Could you check a few things on this drawing? It's one solid part, dimensions in mm from its lowest x, y, z. A direction names the side the tool comes from. Coordinates: 2 decimals unless noted, no trailing zeros. Loops run counter-clockwise (first coordinate to the right, second up) from the corner with the lowest first, then second, coordinate; pieces in that order, holes last.
1) Imagine slicing it at C-C on y = 39. Please give me the cut outline in (x, z), plus the area to 3 significant figures.
2) Will these pins go through, and if not, where does the flat tip stop? P1, Ø7, axis at y = 50, z = 15, coming from the +X side; P2, Ø10, axis at x = 19.5, z = 7, coming from the +Y side; P3, Ø14.5, axis at x = 15, y = 15, coming from the -Z side; P4, Ø12, axis at x = 14.5, z = 9, coming from the +Y side.
3) Imagine slicing it at A-A on z = 15. Please give me the cut outline in (x, y), plus the area to 3 significant figures.
4) Imagine slicing it at D-D on z = 2.25. Please give me the cut outline in (x, y), plus the area to 3 significant figures.
5) Imagine slicing it at B-B on x = 15. Please give me the cut outline in (y, z), plus the area to 3 significant figures.
6) Thinking about a two-plate mould opening in Z: for the marked faces 1, 2, 3 and 4, which applies, released by +Z, released by -Z, zero draft, split by the parting line, or undercut?
7) For the marked faces 5 and 6, which set-ups out of +Z, -Z, +X, -X, +Y, -Y let a thin tool reach every point of the face, with its end or its side?
8) If I drill on line 1 along X through (y, z) = (54, 8.5); line 2 along Z through (x, y) = (2.5, 50); line 3 along Y through (x, z) = (16.5, 22.75), over which ranges is the centre line in solid material (lowest first)?
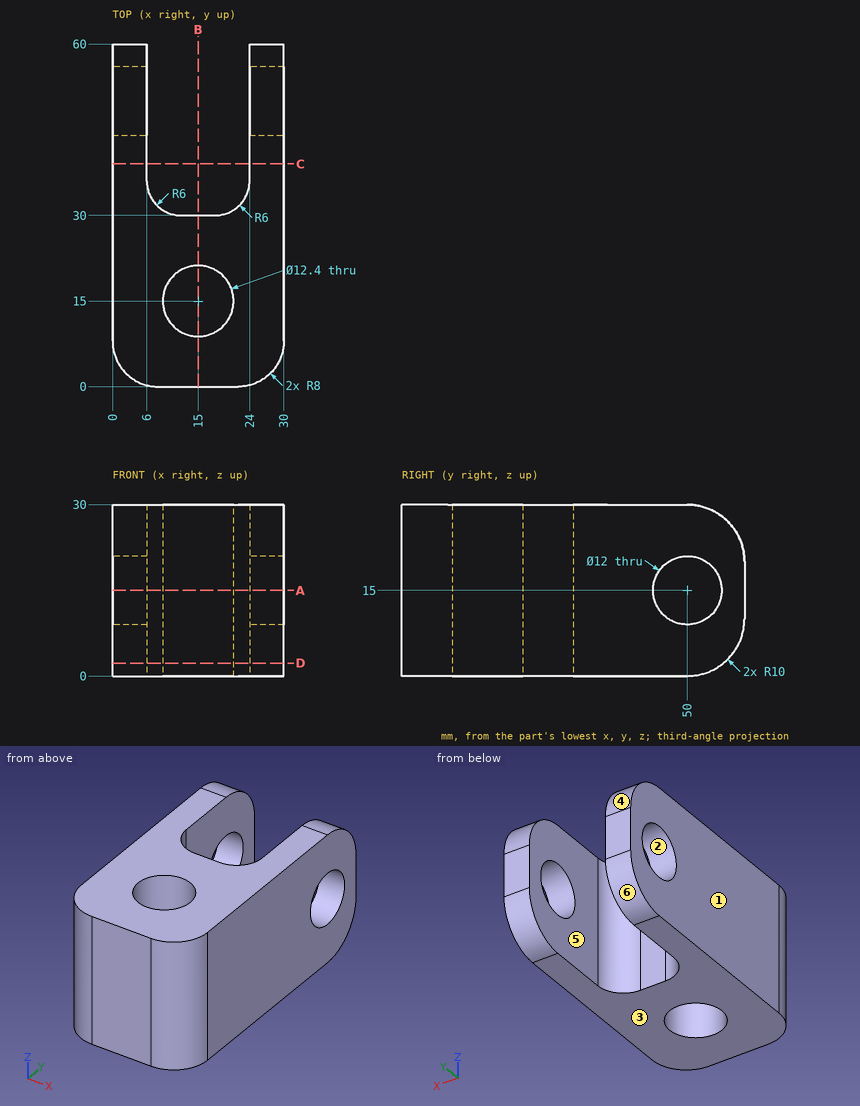
Filled in:
1. outline: (0, 0) - (6, 0) - (6, 30) - (0, 30) - close; (24, 0) - (30, 0) - (30, 30) - (24, 30) - close
1. area: 360 mm2
2. P1: passes through
2. P2: stops at y = 59.97
2. P3: stops at z = 0
2. P4: stops at y = 31.13
3. outline: (0, 8) arc R8 ccw to (8, 0) - (22, 0) arc R8 ccw to (30, 8) - (30, 44) - (24, 44) - (24, 36) arc R6 cw to (18, 30) - (12, 30) arc R6 cw to (6, 36) - (6, 44) - (0, 44) - close; (0, 56) - (6, 56) - (6, 60) - (0, 60) - close; (24, 56) - (30, 56) - (30, 60) - (24, 60) - close; hole circle Ø12.4 at (15, 15)
3. area: 983 mm2
4. outline: (0, 8) arc R8 ccw to (8, 0) - (22, 0) arc R8 ccw to (30, 8) - (30, 56.32) - (24, 56.32) - (24, 36) arc R6 cw to (18, 30) - (12, 30) arc R6 cw to (6, 36) - (6, 56.32) - (0, 56.32) - close; hole circle Ø12.4 at (15, 15)
4. area: 1,080 mm2
5. outline: (0, 0) - (8.8, 0) - (8.8, 30) - (0, 30) - close; (21.2, 0) - (30, 0) - (30, 30) - (21.2, 30) - close
5. area: 528 mm2
6. face 1: zero draft
6. face 2: undercut
6. face 3: released by -Z
6. face 4: released by +Z
7. face 5: +Z, -Z, +Y
7. face 6: -Z, +X, -X, +Y
8. line 1: x = 0 to 6, 24 to 30
8. line 2: z = 0 to 9, 21 to 30
8. line 3: y = 0 to 8.98, 21.02 to 30
